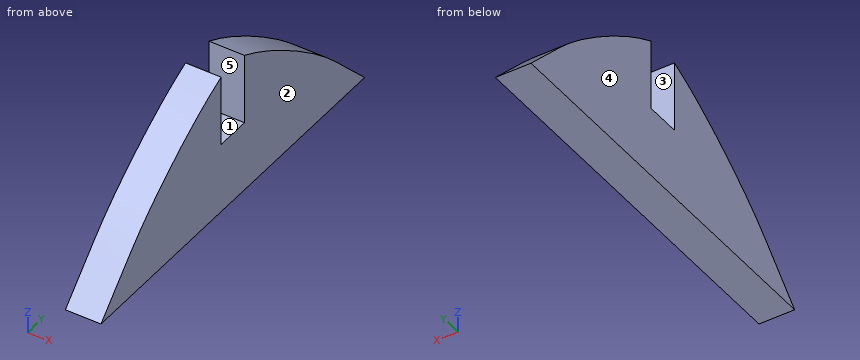
from build123d import *

# Parameters (mm, degrees)
F1_DEPTH = 38.1


with BuildPart() as f1:
    # F0 (on Right) → F1 (new body)
    with BuildSketch(Plane.YZ):
        with BuildLine():
            add(Edge.make_bspline(
                [(-132.4336230755, 0), (-83.8873000655, 49.9797638867), (-61.4657106946, 74.5330828615), (22.5918702379, 134.2773763467), (64.0371870756, 152.4)],
                knots=[0, 0, 0, 0, 0.4863937211, 1, 1, 1, 1], degree=3))
            Line((-132.4336230755, 0), (83.0871870756, 0))
            Line((83.0871870756, 0), (298.6079972267, 0))
            add(Edge.make_bspline(
                [(298.6079972267, 0), (250.0616742167, 49.9797638867), (227.6400848458, 74.5330828615), (143.5825039133, 134.2773763467), (102.1371870756, 152.4)],
                knots=[0, 0, 0, 0, 0.4863937211, 1, 1, 1, 1], degree=3))
            Line((102.1371870756, 152.4), (102.1371870756, 76.1232599616))
            Line((102.1371870756, 76.1232599616), (83.0871870756, 76.1232599616))
            Line((83.0871870756, 76.1232599616), (64.0371870756, 76.1232599616))
            Line((64.0371870756, 76.1232599616), (64.0371870756, 152.4))
        make_face()
    extrude(amount=F1_DEPTH)


solid = f1.part
Geometry: final body of the model. Coordinates: model frame, mm. Face numbers are marked on the shaded views. A direction names the side the tool comes from. Give positions to 0.01 mm unless a question says otherwise; leave off trailing zeros. Use CSV: the item, a comma, the result in double quotes.
1. Material intervals for line 1 along Y through (x, z) = (31, 79); line 2 along Y through (x, z) = (22.5, 37); line 3 along Z through (x, y) = (19.5, 157), sorted ascending. Write a range as from..to.
Answers below:
line 1,"-51.47..64.04, 102.14..217.64"
line 2,"-96.48..262.65"
line 3,"0..122.61"
2. Mould query, pull axis Y, two halves, no side actions, for the marked faces 1, 2 and 3. Classes: +Y half, -Y half, draft (parallel to the pull), parting line (faces both ways), or undercut.
Answers below:
face 1,"undercut"
face 2,"draft"
face 3,"undercut"
3. Contact query for flat-ended pins moving along their axis: pin 1 (2 mm diameter, centred on x = 17.5, y = 11, fed in from -Z); pin 2 (19 mm diameter, centred on x = 27.5, z = 98.5, fed in from +Y); pin 3 (1 mm diameter, centred on x = 5, y = 52, fed in from +Z); pin 4 (8 mm diameter, centred on x = 24.5, y = -21, fed in from +Z). Output: stop coordinate, or through.
Answers below:
pin 1,"z = 0"
pin 2,"y = 204.95"
pin 3,"z = 147.06"
pin 4,"z = 105.05"
4. Access query for the marked faces 4 and 5. Directions: +Z, -Z, +X, -X, +Y, -Y. A direction counts if a zero-diameter tool reaches every point of the face in a straight line with its end or side. Return the directions, or none.
Answers below:
face 4,"+Z, -Z, -X, +Y, -Y"
face 5,"+Z, +X, -X"
